The listing builds one solid part. Answer for the finished solid, in the listing's coordinates (mm). A direction names the side the tool comes from. Coordinates: 2 decimals unless noted, no trailing zeros. Order: outer loops, then holes, each group sorted by start corner. A loop starts at its lowest first (then second) coordinate and runs counter-clockwise, first axis right, second up. Notation, with made-up numbers: (77.25, -37) - (131.25, -37) arc R13 cw to (131.25, -32) - close; hole circle Ø6 at (-30.75, 64.5). An arc over 180 degrees is marked (long way). Use a Markdown table: item, result. Add a question column.
Item 1: The part is cut by section C-C, the plane z = -10. Give the vertices of the cut face in (x, y).
Item 2: For faces 5 (the flat face through (-13, 2, -48)), 6 (the flat face through (9.5, 3, -4)), determine the directions among +Z, -Z, +X, -X, +Y, -Y from which every point of the face is accessible in a straight line to the end or side of a thin tool.
Item 3: The part is cut by section B-B, the plane y = 3.25. Give the vertices of the cut face in (x, z), then the cut area to 3 significant figures.
Item 4: Find the intervals of material crossed by line 1 along X through (y, z) = (4.5, -5); line 2 along Z through (x, y) = (-20.5, 0.25); line 3 along X through (y, z) = (3.25, -4), in increasing order.
Item 5: The mould has two halves that part along Z. Classify faces 1 (the flat face through (6, 3, -12)), 2 (the flat face through (-13, 5, -11)), 3 (the flat face through (-13, 2, 3)), 4 (the flat face through (-28.5, 5, -34)): released by +Z, released by -Z, zero draft, split by the parting line, or undercut.
Item 6: The part is cut by section D-D, the plane y = 6.25. Give the vertices of the cut face in (x, z), then the cut area to 3 significant figures.
Item 7: Flat-ended cylindrical pins translate along their axes: P1, Ø2, axis at x = 5, z = -8, coming from the -Y side; P2, Ø4, axis at y = -2, z = -19, coming from the -X side; P3, Ø2.5, axis at y = 2.5, z = -41.5, coming from the +X side. Find the tip coordinate at first contact, or state that the pin passes through.
Item 8: The part is cut by section A-A, the plane x = 5. Give the vertices of the cut face in (y, z), then the cut area to 3 significant figures.
from build123d import *

# Parameters (mm, degrees)
SKETCH1_W           = 26
SKETCH1_H           = 53
SKETCH1_W_2         = 20
SKETCH1_H_2         = 10
BOSS_EXTRUDE1_DEPTH = 5
SKETCH2_W           = 31
SKETCH2_H           = 59
SKETCH2_W_2         = 26
SKETCH2_H_2         = 53
BOSS_EXTRUDE2_DEPTH = 10
SKETCH3_W           = 31
SKETCH3_H           = 59
BOSS_EXTRUDE3_DEPTH = 3
CHAMFER1_SIZE       = 0.5
CHAMFER1_SIZE2      = 7.150333128
SKETCH10_W          = 7
SKETCH10_H          = 15
SKETCH10_R          = 2.25
BOSS_EXTRUDE7_DEPTH = 10


with BuildPart() as part:
    # Sketch1 → Boss-Extrude1 (new body)
    with BuildSketch(Plane(origin=(0, 0, 0), x_dir=(1, 0, 0), z_dir=(0, 1, 0))):
        with Locations((-13, 26.5)):
            Rectangle(SKETCH1_W, SKETCH1_H)
        with Locations((-13, 27)):
            Rectangle(SKETCH1_W_2, SKETCH1_H_2, mode=Mode.SUBTRACT)
        with Locations((-13, 43)):
            Rectangle(SKETCH1_W_2, SKETCH1_H_2, mode=Mode.SUBTRACT)
        with Locations((-13, 11)):
            Rectangle(SKETCH1_W_2, SKETCH1_H_2, mode=Mode.SUBTRACT)
    extrude(amount=BOSS_EXTRUDE1_DEPTH)

    # Sketch2 → Boss-Extrude2 (add)
    with BuildSketch(Plane(origin=(0, 5, 0), x_dir=(1, 0, 0), z_dir=(0, 1, 0))):
        with Locations((-13, 26.5)):
            Rectangle(SKETCH2_W, SKETCH2_H)
        with Locations((-13, 26.5)):
            Rectangle(SKETCH2_W_2, SKETCH2_H_2, mode=Mode.SUBTRACT)
    extrude(amount=-BOSS_EXTRUDE2_DEPTH)

    # Sketch3 → Boss-Extrude3 (add)
    with BuildSketch(Plane(origin=(0, 5, 0), x_dir=(1, 0, 0), z_dir=(0, 1, 0))):
        with Locations((-13, 26.5)):
            Rectangle(SKETCH3_W, SKETCH3_H)
    extrude(amount=BOSS_EXTRUDE3_DEPTH)

    # Chamfer1
    chamfer1_edges = [part.edges().sort_by_distance(p)[0] for p in [
        (-28.5, -5, -26.5),
        (2.5, -5, -26.5),
    ]]
    chamfer1_side = [part.faces().sort_by_distance(p)[0] for p in [
        (-13, -5, -55.333516692),
    ]]
    chamfer(chamfer1_edges, length=CHAMFER1_SIZE, length2=CHAMFER1_SIZE2, reference=chamfer1_side[0])

    # Sketch10 → Boss-Extrude7 (add)
    with BuildSketch(Plane(origin=(0, 8, 0), x_dir=(1, 0, 0), z_dir=(0, 1, 0))):
        with Locations((6, 4.5)):
            Rectangle(SKETCH10_W, SKETCH10_H)
        with Locations((5, 5)):
            Circle(SKETCH10_R, mode=Mode.SUBTRACT)
        with Locations((-32, 4.5)):
            Rectangle(SKETCH10_W, SKETCH10_H)
        with Locations((-31, 5)):
            Circle(SKETCH10_R, mode=Mode.SUBTRACT)
    extrude(amount=-BOSS_EXTRUDE7_DEPTH)


solid = part.part
Solution:
| question | item | result |
|---|---|---|
| 1 | outline | (-35.5, -2) - (-28.5, -2) - (-28.5, 2.15) - (-28, -5) - (-26, -5) - (-26, 0) - (-23, 0) - (-23, 5) - (-3, 5) - (-3, 0) - (0, 0) - (0, -5) - (2, -5) - (2.5, 2.15) - (2.5, -2) - (9.5, -2) - (9.5, 8) - (-35.5, 8) - close |
| 2 | face 5 | -Y |
| 2 | face 6 | +Z, -Z, +X, +Y, -Y |
| 3 | outline | (-35.5, -12) - (-28.5, -12) - (-28.5, -56) - (2.5, -56) - (2.5, -12) - (9.5, -12) - (9.5, 3) - (-35.5, 3) - close; hole circle Ø4.5 at (-31, -5); hole (-23, -48) - (-3, -48) - (-3, -38) - (-23, -38) - close; hole (-23, -32) - (-3, -32) - (-3, -22) - (-23, -22) - close; hole (-23, -16) - (-3, -16) - (-3, -6) - (-23, -6) - close; hole circle Ø4.5 at (5, -5) |
| 3 | area | 1,410 mm2 |
| 4 | line 1 | x = -35.5 to -33.25, -28.75 to 2.75, 7.25 to 9.5 |
| 4 | line 2 | z = -56 to -48, -38 to -32, -22 to -16, -6 to 3 |
| 4 | line 3 | x = -35.5 to -33.02, -28.98 to 2.98, 7.02 to 9.5 |
| 5 | face 1 | released by -Z |
| 5 | face 2 | undercut |
| 5 | face 3 | released by +Z |
| 5 | face 4 | zero draft |
| 6 | outline | (-35.5, -12) - (-28.5, -12) - (-28.5, -56) - (2.5, -56) - (2.5, -12) - (9.5, -12) - (9.5, 3) - (-35.5, 3) - close; hole circle Ø4.5 at (-31, -5); hole circle Ø4.5 at (5, -5) |
| 6 | area | 2,010 mm2 |
| 7 | P1 | stops at y = -2 |
| 7 | P2 | stops at x = -28.35 |
| 7 | P3 | stops at x = 2.5 |
| 8 | outline | (-2, -12) - (8, -12) - (8, -7.25) - (-2, -7.25) - close; (-2, -2.75) - (8, -2.75) - (8, 3) - (-2, 3) - close |
| 8 | area | 105 mm2 |
